Geometry check sheet. Reference: the model listing, model coordinates, mm. A direction names the side the tool comes from. Coordinates: 2 decimals unless noted, no trailing zeros. Write each loop counter-clockwise with the first axis right and the second up, starting at its lowest first coordinate (ties: lowest second). Pieces come first, ordered by that corner, then holes. Notation, with made-up numbers: M 20,18.5 L 78,18.5 A35 cw 78,54.5 Z; hole C 23,-26.5 d8. An arc over 180 degrees is marked long. Write each question's results on one line, items separated by ' | '.
Autodesk Inventor part; units mm, degrees
ref_plane "YZ Plane" through (0, 0, 0) normal (1, 0, 0) x (0, 1, 0)
ref_plane "XZ Plane" through (0, 0, 0) normal (0, 1, 0) x (-1, 0, 0)
ref_plane "XY Plane" through (0, 0, 0) normal (0, 0, 1) x (1, 0, 0)
sketch "スケッチ1" plane through (0, 0, 0) normal (0, 0, 1) x (1, 0, 0)
  circle A0 centre (0, 0) radius 48.5
  circle A1 centre (0, 0) radius 46.0893
  line L0 (-50, 50) -> (50, 50)
  line L1 (50, 50) -> (50, -50)
  line L2 (50, -50) -> (-50, -50)
  line L3 (-50, -50) -> (-50, 50)
  dimension "d0" = 97
  dimension "d3" = 50
  dimension "d4" = 50
  dimension "d5" = 50
  dimension "d6" = 50
extrude "押し出し1" add sketch "スケッチ1" along normal blind 5 contours A0 | A1 | L0 L1 L2 L3
sketch "スケッチ2" plane through (0, 0, 5) normal (0, 0, 1) x (1, 0, 0)
  circle A0 centre (0, 0) radius 46
  line L0 (0, 0) -> (0, 64.6511)
  line L1 (0, 0) -> (-25.9524, 62.6547)
  line L2 (-50, 50) -> (-50, -50)
  point P0 (-17.6034, 42.4985)
  point P1 (-42.4985, 17.6034)
  point P2 (-42.4985, -17.6034)
  point P3 (-17.6034, -42.4985)
  point P4 (17.6034, -42.4985)
  point P5 (42.4985, -17.6034)
  point P6 (42.4985, 17.6034)
  point P7 (17.6034, 42.4985)
  dimension "d7" = 92
  dimension "d8" = 22.5
  dimension "d11" = 360
  dimension "d76" = 50
hole "穴1" at (-17.6034, 42.4985, 5) at (-42.4985, 17.6034, 5) at (-42.4985, -17.6034, 5) at (-17.6034, -42.4985, 5) at (17.6034, -42.4985, 5) at (42.4985, -17.6034, 5) at (42.4985, 17.6034, 5) at (17.6034, 42.4985, 5) direction (0, 0, -1) diameter 2.459 end through all
sketch "スケッチ3" plane through (0, 0, 5) normal (0, 0, 1) x (1, 0, 0)
  circle A0 centre (0, 0) radius 30
  dimension "d20" = 60
extrude "押し出し2" cut sketch "スケッチ3" against normal blind 5
sketch "スケッチ4" plane through (50, -50, 0) normal (1, 0, 0) x (0, 0, -1)
  line L0 (-5, 100) -> (-5, 0)
  line L1 (-5, 100) -> (0, 100)
  line L2 (0, 100) -> (0, 0)
  line L3 (0, 0) -> (-5, 0)
  line L4 (-5, 0) -> (-5, 100)
  point P0 (0, 50)
extrude "押し出し3" add sketch "スケッチ4" along normal blind 40
sketch "スケッチ5" plane through (0, 0, 5) normal (0, 0, 1) x (1, 0, 0)
  line L0 (-50, 50) -> (90, 50)
  line L1 (85, 50) -> (90, 50)
  line L2 (90, 50) -> (90, -50)
  line L3 (90, -50) -> (85, -50)
  line L4 (85, -50) -> (85, 50)
  line L5 (-50, -50) -> (90, -50)
  line L6 (90, 50) -> (90, -50)
  point P0 (0, 0)
  point P1 (90, 50)
  point P2 (90, 0)
  dimension "d25" = 0
  dimension "d26" = 5
  dimension "d27" = 100
  dimension "d70" = 0
extrude "押し出し4" add sketch "スケッチ5" along normal blind 100
sketch "スケッチ6" plane through (90, -50, 0) normal (1, 0, 0) x (0, 0, -1)
  circle A0 centre (-55, 50) radius 46
  line L0 (0, 0) -> (-105, 0)
  line L1 (0, 0) -> (0, 100)
  line L2 (-55, 50) -> (41.9537, 50)
  line L3 (-55, 50) -> (-55, 131.7305)
  line L4 (-55, 50) -> (-80.0101, 110.3797)
  circle A1 centre (-55, 50) radius 12.5
  line L5 (-55, 50) -> (-63.1841, 64.1753)
  point P0 (0, 50)
  point P1 (-72.6034, 92.4985)
  point P2 (-97.4985, 67.6034)
  point P3 (-97.4985, 32.3966)
  point P4 (-72.6034, 7.5015)
  point P5 (-37.3966, 7.5015)
  point P6 (-12.5015, 32.3966)
  point P7 (-12.5015, 67.6034)
  point P8 (-37.3966, 92.4985)
  point P9 (-61.25, 60.8253)
  point P10 (-67.5, 50)
  point P11 (-61.25, 39.1747)
  point P12 (-48.75, 39.1747)
  point P13 (-42.5, 50)
  point P14 (-48.75, 60.8253)
  dimension "d32" = 92
  dimension "d34" = 25
  dimension "d30" = 50
  dimension "d31" = 55
  dimension "d33" = 22.5
  dimension "d35" = 30
  dimension "d38" = 360
  dimension "d42" = 360
hole "穴2" at (90, 42.4985, 72.6034) at (90, 17.6034, 97.4985) at (90, -17.6034, 97.4985) at (90, -42.4985, 72.6034) at (90, -42.4985, 37.3966) at (90, -17.6034, 12.5015) at (90, 17.6034, 12.5015) at (90, 42.4985, 37.3966) at (90, 10.8253, 61.25) at (90, 0, 67.5) at (90, -10.8253, 61.25) at (90, -10.8253, 48.75) at (90, 0, 42.5) at (90, 10.8253, 48.75) direction (-1, 0, 0) diameter 2.459 end through all
sketch "スケッチ7" plane through (90, -50, 0) normal (1, 0, 0) x (0, 0, -1)
  line L0 (-55, 50) -> (26.223, 50)
  circle A0 centre (-55, 50) radius 10.2
  line L1 (0, 0) -> (0, 100)
  line L2 (0, 0) -> (-105, 0)
  line L3 (-55, 50) -> (-55, 82.0983)
  point P0 (0, 50)
  point P1 (-55, 60.2)
  point P2 (-63.8335, 44.9)
  point P3 (-46.1665, 44.9)
  dimension "d53" = 20.4
  dimension "d51" = 55
  dimension "d52" = 50
  dimension "d56" = 360
hole "穴3" at (90, 10.2, 55) at (90, -5.1, 63.8335) at (90, -5.1, 46.1665) direction (-1, 0, 0) diameter 4 end through all
sketch "スケッチ8" plane through (90, -50, 0) normal (1, 0, 0) x (0, 0, -1)
  circle A0 centre (-55, 50) radius 6.5
  line L0 (0, 0) -> (0, 100)
  line L1 (0, 0) -> (-105, 0)
  point P0 (0, 50)
  dimension "d65" = 13
  dimension "d66" = 55
  dimension "d67" = 50
extrude "押し出し5" cut sketch "スケッチ8" against normal through all
properties part number "legparts_07"
Q1. Sectioned sample at C-C on x = 62.5. Record the cut outline in (y, z), and give its area (3 significant figures).
Geometry check:
outline: M -50,0 L 50,0 L 50,5 L -50,5 Z | area: 500 mm2
Q2. Sectioned sample at B-B on z = 32.5. Record the cut outline in (x, y), and give its area (3 significant figures).
Geometry check:
outline: M 85,-50 L 90,-50 L 90,50 L 85,50 Z | area: 500 mm2
Q3. Scan lines: probe 1 along Z at (x, y) = (86.75, 10.2); probe 2 along X at (y, z) = (43, 92.5); probe 3 along Y at (x, z) = (88.65, 42.5). Record each from-to range of solid material in increasing order.
Geometry check:
probe 1: z = 0 to 47.69, 49.81 to 53, 57 to 60.19, 62.31 to 105 | probe 2: x = 85 to 90 | probe 3: y = -50 to -1.23, 1.23 to 50
Q4. Mould release check, pull along Z, two halves, no side actions. Record for faces 3 (the cylindrical face through (87.5, -4.3, 62)), 4 (the flat face through (87, 1, 105)), 5 (the flat face through (51, -50, 2)), 6 (the cylindrical face through (87.54, 1.95, 48.8)): pulls with the +Z half, pulls with the -Z half, needs draft (parallel to the pull), parting line crosses it, or undercut.
Geometry check:
face 3: undercut | face 4: pulls with the +Z half | face 5: needs draft | face 6: undercut
Q5. Depth check by flat-ended pin: P1, Ø2, axis at y = 42.5, z = 37.4, coming from the -X side; P2, Ø10, axis at x = 70.5, y = -9.5, coming from the -Z side; P3, Ø4, axis at y = 17.6, z = 12.5, coming from the -X side; P4, Ø3, axis at x = -2, y = 35.5, coming from the +Z side. Enter the tip coordinate at first touch or a pass-through.
Geometry check:
P1: passes through | P2: stops at z = 0 | P3: stops at x = 85 | P4: stops at z = 5
Q6. Access from +Z, -Z, +X, -X, +Y, -Y to the whole of each face (thin tool, end or side, straight path). Record for faces 1 (the flat face through (32, 1, 5)), 2 (the flat face through (35, 1, 0)).
Geometry check:
face 1: +Z, -X, +Y, -Y | face 2: -Z, +X, -X, +Y, -Y
Q7. Sectioned sample at A-A on x = 3. Record the cut outline in (y, z).
Geometry check:
outline: M -50,0 L -29.85,0 L -29.85,5 L -50,5 Z; M 29.85,0 L 50,0 L 50,5 L 29.85,5 Z
